```python
from build123d import *

# Parameters (mm, degrees)
PAD_DEPTH       = 2
SKETCH001_W     = 30
SKETCH001_H     = 70
PAD001_DEPTH    = 2
PAD002_DEPTH    = 2
PAD003_DEPTH    = 2
POCKET_DEPTH    = 2
SKETCH005_W     = 16
SKETCH005_H     = 58
POCKET001_DEPTH = 2
FILLET_R        = 1
FILLET001_R     = 1


with BuildPart() as part:
    # Sketch → Pad (new body)
    with BuildSketch(Plane.XY):
        with BuildLine():
            Line((-15, -5), (-15, 15))
            Line((-15, 15), (15, 15))
            Line((15, 15), (15, -5))
            ThreePointArc((-15, -5), (0, -20), (15, -5))
        make_face()
    extrude(amount=PAD_DEPTH)

    # Sketch001 (on Face2 of Pad) → Pad001 (join)
    with BuildSketch(Plane(origin=(0, 15, 0), x_dir=(-1, 0, 0), z_dir=(0, 1, 0))):
        with Locations((0, 37)):
            Rectangle(SKETCH001_W, SKETCH001_H)
    extrude(amount=-PAD001_DEPTH)

    # Sketch002 (on Face11 of Pad001) → Pad002 (join)
    with BuildSketch(Plane.YZ.offset(15)):
        Polygon((13, 72), (13, 2), (-5, 2), align=None)
    pad002 = extrude(amount=-PAD002_DEPTH)

    # Mirrored: Pad002 across YZ
    add(pad002.mirror(Plane.YZ))

    # Sketch003 (on Face11 of Mirrored) → Pad003 (join)
    with BuildSketch(Plane.XY.offset(72)):
        with BuildLine():
            Line((-13, 13), (13, 13))
            Line((13, 13), (13, 8))
            ThreePointArc((-13, 8), (0, -5), (13, 8))
            Line((-13, 13), (-13, 8))
        make_face()
    extrude(amount=-PAD003_DEPTH)

    # Sketch004 (on Face19 of Pad003) → Pocket (cut)
    with BuildSketch(Plane.XY.offset(72)):
        with BuildLine():
            ThreePointArc((3.832963, 4.164), (0, 10.25), (-3.832963, 4.164))
            add(Edge.make_bspline(
                [(-3.832963, 4.164), (-3, 1.5), (-3.5, -4.519984)],
                knots=[0, 0, 0, 1, 1, 1], degree=2))
            ThreePointArc((-3.5, -4.519984), (0, -5), (3.5, -4.519984))
            add(Edge.make_bspline(
                [(3.832963, 4.164), (3, 1.5), (3.5, -4.519984)],
                knots=[0, 0, 0, 1, 1, 1], degree=2))
        make_face()
    extrude(amount=-POCKET_DEPTH, mode=Mode.SUBTRACT)

    # Sketch005 (on Face17 of Pocket) → Pocket001 (cut)
    with BuildSketch(Plane.XZ.offset(-13)):
        with Locations((0, 36)):
            Rectangle(SKETCH005_W, SKETCH005_H)
    extrude(amount=-POCKET001_DEPTH, mode=Mode.SUBTRACT)

    # Fillet
    fillet_edges = [part.edges().sort_by_distance(p)[0] for p in [
        (-3.31397, -0.158011, 72),
        (0, 10.25, 72),
        (3.31397, -0.158011, 72),
    ]]
    fillet(fillet_edges, radius=FILLET_R)

    # Fillet001
    fillet001_edges = [part.edges().sort_by_distance(p)[0] for p in [
        (-8, 14, 7),
        (8, 14, 7),
        (8, 14, 65),
        (-8, 14, 65),
    ]]
    fillet(fillet001_edges, radius=FILLET001_R)


solid = part.part
```
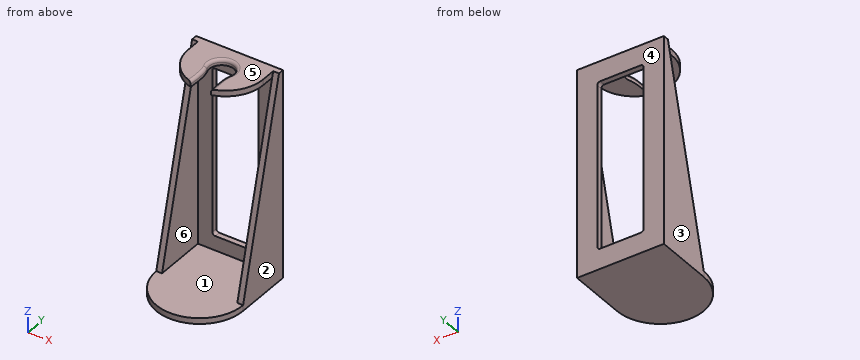
Model file for the job. Use its own axes, mm. Face numbers are marked on the shaded views. A direction names the side the tool comes from. Coordinates: 2 decimals unless noted, no trailing zeros. Order: outer loops, then holes, each group sorted by start corner. A loop starts at its lowest first (then second) coordinate and runs counter-clockwise, first axis right, second up. Notation, with made-up numbers: (72, -2) -> (79, -2) arc R29 ccw to (79, 32) -> close; hole circle Ø7 at (22.25, 42). An arc over 180 degrees is marked (long way). Answer as a JSON object with one key per item and string values. Group by question number.
1) Cut at A-A, the plane x = 0. Write the cut outline in (y, z), then the cut area to 3 significant figures.
2) Cut at C-C, the plane x = -12. Write the cut outline in (y, z), then the cut area to 3 significant figures.
3) Pull direction X, two halves, no side cores. Call the marked faces 1, 2, 3 and 4: +X half, -X half, draft (parallel to the pull), parting line (faces both ways), or undercut.
4) Which spindle directions (+Z, -Z, +X, -X, +Y, -Y) get a long thin tool onto all of the face, cutting with end or side? Do the marked faces 5 and 6. Say none if no direction does.
5) Cut at D-D, the plane y = -2.5. Count the separate pieces of the cut face and the enclosed holes in it, then the cut area to 3 significant figures.
6) Cut at B-B, the plane z = 17. Write the cut outline in (x, y).
7) Drill centre lines: L1, parallel to X at y = 6.5, z = 31; L2, parallel to Z at x = 9, y = 5; L3, parallel to Z at x = 13, y = -10. Where is each one in solid material? Low to high.
8) Flat gauge pins, fed straight in: pin 1 (5 mm diameter, centred on x = -2.5, y = -15.5, fed in from +Z); pin 2 (2 mm diameter, centred on y = 11.5, z = 71.5, fed in from +X); pin 3 (2 mm diameter, centred on y = 11, z = 71.5, fed in from -X). Where does each tip first touch, or does it go through?
Check values:
{
 "1": {"outline": "(-20, 0) -> (15, 0) -> (15, 7) -> (13, 7) -> (13, 2) -> (-20, 2) -> close; (10.25, 70) -> (13, 70) -> (13, 65) -> (15, 65) -> (15, 72) -> (11.25, 72) arc R1 ccw to (10.25, 71) -> close", "area": "99.3 mm²"},
 "2": {"outline": "(-14, 0) -> (15, 0) -> (15, 72) -> (3, 72) -> (3, 70) -> (13, 70) -> (13, 2) -> (-14, 2) -> close", "area": "218 mm²"},
 "3": {"face 1": "undercut", "face 2": "+X half", "face 3": "-X half", "face 4": "draft"},
 "4": {"face 5": "+Z, +X, -X, +Y, -Y", "face 6": "-Y"},
 "5": {"separate pieces": "3", "enclosed holes": "0", "area": "116 mm²"},
 "6": {"outline": "(-15, -1.14) -> (-13, -1.14) -> (-13, 13) -> (-8, 13) -> (-8, 15) -> (-15, 15) -> close; (8, 13) -> (13, 13) -> (13, -1.14) -> (15, -1.14) -> (15, 15) -> (8, 15) -> close"},
 "7": {"L1": "x = -15 to -13, 13 to 15", "L2": "z = 0 to 2, 70 to 72", "L3": "z = 0 to 2"},
 "8": {"pin 1": "stops at z = 2", "pin 2": "stops at x = 13", "pin 3": "stops at x = -13"}
}
